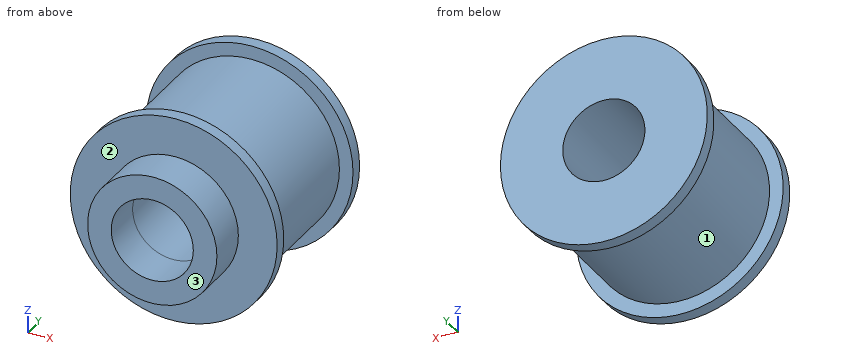
from build123d import *

# Parameters (mm, degrees)
SKETCH1_R               = 13.9
BOSS_EXTRUDE1_DEPTH     = 21
SKETCH2_R               = 16
BOSS_EXTRUDE2_DEPTH     = 2
SKETCH3_R               = 16
BOSS_EXTRUDE3_DEPTH     = 2
SKETCH5_R               = 10
SKETCH5_R_2             = 3
BOSS_EXTRUDE4_DEPTH     = 6.5
SKETCH4_R               = 6.35
CUT_EXTRUDE1_DEPTH      = 10
CUT_EXTRUDE1_DEPTH_BACK = 26


with BuildPart() as part:
    # Sketch1 → Boss-Extrude1 (new body)
    with BuildSketch(Plane(origin=(0, 0, 0), x_dir=(1, 0, 0), z_dir=(0, 1, 0))):
        Circle(SKETCH1_R)
    extrude(amount=BOSS_EXTRUDE1_DEPTH)

    # Sketch2 → Boss-Extrude2 (add)
    with BuildSketch(Plane(origin=(0, 21, 0), x_dir=(1, 0, 0), z_dir=(0, 1, 0))):
        Circle(SKETCH2_R)
    extrude(amount=BOSS_EXTRUDE2_DEPTH)

    # Sketch3 → Boss-Extrude3 (add)
    with BuildSketch(Plane.XZ):
        Circle(SKETCH3_R)
    extrude(amount=BOSS_EXTRUDE3_DEPTH)

    # Sketch5 → Boss-Extrude4 (add)
    with BuildSketch(Plane.XZ.offset(2)):
        Circle(SKETCH5_R)
        Circle(SKETCH5_R_2, mode=Mode.SUBTRACT)
    extrude(amount=BOSS_EXTRUDE4_DEPTH)

    # Sketch4 → Cut-Extrude1 (cut, two sides)
    with BuildSketch(Plane.XZ.offset(2)) as cut_extrude1_sk:
        Circle(SKETCH4_R)
    extrude(amount=CUT_EXTRUDE1_DEPTH, mode=Mode.SUBTRACT)
    extrude(cut_extrude1_sk.sketch, amount=-CUT_EXTRUDE1_DEPTH_BACK, mode=Mode.SUBTRACT)


solid = part.part
Design review of the part built by this model. Coordinates are the model's own, in mm. Face numbers are marked on the shaded views. A direction names the side the tool comes from. Coordinates: 2 decimals unless noted, no trailing zeros. Order: outer loops, then holes, each group sorted by start corner. A loop starts at its lowest first (then second) coordinate and runs counter-clockwise, first axis right, second up. Notation, with made-up numbers: M 12,-14.5 L 25,-14.5 A10 cw 25,0.5 Z; hole C -10,43 d2. An arc over 180 degrees is marked long. Use a Markdown table: item, result.
(1) Wall thickness on probe 1 along Z at (x, y) = (0, 10.25); probe 2 along Y at (x, z) = (-10, 11); probe 3 along Z at (x, y) = (0, -5): over which ranges is each line inside the solid? List them lowest first.
Worked answers:
| item | result |
|---|---|
| probe 1 | z = -13.9 to -6.35, 6.35 to 13.9 |
| probe 2 | y = -2 to 0, 21 to 23 |
| probe 3 | z = -10 to -6.35, 6.35 to 10 |
(2) For P1, Ø1, axis at x = 0.5, y = -4, coming from the +Z side; P2, Ø10, axis at x = 0, z = 0, coming from the -Y side; P3, Ø14.5, axis at x = 0, z = 0, coming from the +Y side; P4, Ø2, axis at y = 4, z = 11.5, coming from the +X side, all flat-tipped, find the tip position at first contact; note any pin that passes through.
Worked answers:
| item | result |
|---|---|
| P1 | stops at z = 10 |
| P2 | passes through |
| P3 | stops at y = 23 |
| P4 | stops at x = 9.11 |
(3) Add section C-C (y = -1). Give the boundary of the cut face in (x, z), then the cut area to 3 significant figures.
Worked answers:
| item | result |
|---|---|
| outline | C 0,0 d32; hole C 0,0 d12.7 |
| area | 678 mm2 |
(4) Add section A-A (z = 0). Give the boundary of the cut face in (x, y), then the cut area to 3 significant figures.
Worked answers:
| item | result |
|---|---|
| outline | M -16,-2 L -10,-2 L -10,-8.5 L -6.35,-8.5 L -6.35,23 L -16,23 L -16,21 L -13.9,21 L -13.9,0 L -16,0 Z; M 6.35,-8.5 L 10,-8.5 L 10,-2 L 16,-2 L 16,0 L 13.9,0 L 13.9,21 L 16,21 L 16,23 L 6.35,23 Z |
| area | 442 mm2 |
(5) For the marked faces 1, 2 and 3, list the 3-axis set-ups (+Z, -Z, +X, -X, +Y, -Y) from which the entire face can be reached by the end or side of a thin tool; tool diameter is ignored.
Worked answers:
| item | result |
|---|---|
| face 1 | none |
| face 2 | -Y |
| face 3 | +Z, -Z, +X, -X, -Y |
(6) Add section B-B (x = 0). Give the boundary of the cut face in (y, z), then the cut area to 3 significant figures.
Worked answers:
| item | result |
|---|---|
| outline | M -8.5,-10 L -2,-10 L -2,-16 L 0,-16 L 0,-13.9 L 21,-13.9 L 21,-16 L 23,-16 L 23,-6.35 L -8.5,-6.35 Z; M -8.5,6.35 L 23,6.35 L 23,16 L 21,16 L 21,13.9 L 0,13.9 L 0,16 L -2,16 L -2,10 L -8.5,10 Z |
| area | 442 mm2 |
(7) Add section D-D (x = 11). Give the boundary of the cut face in (y, z), then the cut area to 3 significant figures.
Worked answers:
| item | result |
|---|---|
| outline | M -2,-11.62 L 0,-11.62 L 0,-8.5 L 21,-8.5 L 21,-11.62 L 23,-11.62 L 23,11.62 L 21,11.62 L 21,8.5 L 0,8.5 L 0,11.62 L -2,11.62 Z |
| area | 450 mm2 |
